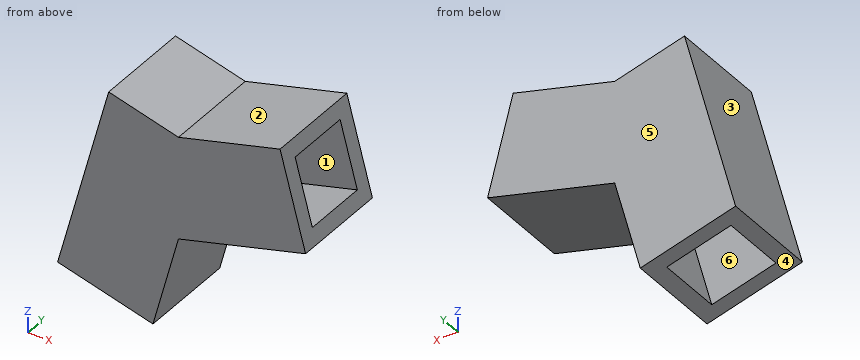
from build123d import *

# Parameters (mm, degrees)
BOSS_EXTRUDE1_DEPTH = 15
SKETCH2_W           = 10.1
SKETCH2_H           = 10.1
CUT_EXTRUDE1_DEPTH  = 18
SKETCH3_W           = 10.1
SKETCH3_H           = 10.1
CUT_EXTRUDE2_DEPTH  = 17
CUT_EXTRUDE3_REACH  = 41.336
SKETCH4_W           = 8
SKETCH4_H           = 8
CUT_EXTRUDE4_REACH  = 34.317
SKETCH5_W           = 8
SKETCH5_H           = 8
FILLET1_R           = 6
FILLET2_R           = 3


with BuildPart() as part:
    # Sketch1 → Boss-Extrude1 (new body)
    with BuildSketch(Plane(origin=(0, 0, 0), x_dir=(1, 0, 0), z_dir=(0, 1, 0))):
        Polygon((0, 0), (15.436230849, -4.13612559), (19.318516526, 10.352761804), (0, 15.529142706), (-3.882285677, 30.0180301), (-18.371173071, 26.135744424), (-10.606601718, -2.842030365), align=None)
    extrude(amount=BOSS_EXTRUDE1_DEPTH)

    # Sketch2 → Cut-Extrude1 (cut)
    with BuildSketch(Plane(origin=(15.436230849, 0, 4.13612559), x_dir=(0.2588190451025214, 0, -0.9659258262890681), z_dir=(0.9659258262890681, 0, 0.2588190451025214))):
        with Locations((7.5, 7.5)):
            Rectangle(SKETCH2_W, SKETCH2_H)
    extrude(amount=-CUT_EXTRUDE1_DEPTH, mode=Mode.SUBTRACT)

    # Sketch3 → Cut-Extrude2 (cut)
    with BuildSketch(Plane(origin=(-7.764571353, 0, -28.977774789), x_dir=(-0.9659258262890682, 0, 0.2588190451025212), z_dir=(-0.2588190451025212, 0, -0.9659258262890682))):
        with Locations((3.480762114, 7.5)):
            Rectangle(SKETCH3_W, SKETCH3_H)
    extrude(amount=-CUT_EXTRUDE2_DEPTH, mode=Mode.SUBTRACT)

    # Cut-Extrude3: up to this plane
    cut_extrude3_end = Plane(origin=(-11.60473103, 12.55, -10.349112038), z_dir=(-0.9659258262890682, 0, 0.2588190451025212))
    # Sketch4 → Cut-Extrude3 (cut, up to the surface)
    with BuildSketch(Plane(origin=(-1.950434024, 0, -0.522617222), x_dir=(0.25881904510252146, 0, -0.9659258262890681), z_dir=(0.9659258262890681, 0, 0.25881904510252146)), mode=Mode.PRIVATE) as cut_extrude3_sk1:
        with Locations((7.5, 7.5)):
            Rectangle(SKETCH4_W, SKETCH4_H)
    cut_extrude3_tool1 = split(extrude(cut_extrude3_sk1.sketch, amount=-CUT_EXTRUDE3_REACH, mode=Mode.PRIVATE), bisect_by=cut_extrude3_end, keep=Keep.BOTH, mode=Mode.PRIVATE)
    add(cut_extrude3_tool1.solids().sort_by_distance((-0.009291, 7.5, -7.767061))[0], mode=Mode.SUBTRACT)

    # Cut-Extrude4: up to this face of the body (flat: up to its plane)
    cut_extrude4_end = Plane(part.part.faces().sort_by_distance((-5.802700436, 7.5, -5.178295527))[0])
    # Sketch5 → Cut-Extrude4 (cut, up to the picked face)
    with BuildSketch(Plane(origin=(-3.364647586, 0, -12.557035742), x_dir=(-0.9659258262890682, 0, 0.25881904510252124), z_dir=(-0.25881904510252124, 0, -0.9659258262890682)), mode=Mode.PRIVATE) as cut_extrude4_sk1:
        with Locations((3.480762114, 7.5)):
            Rectangle(SKETCH5_W, SKETCH5_H)
    cut_extrude4_tool1 = split(extrude(cut_extrude4_sk1.sketch, amount=-CUT_EXTRUDE4_REACH, mode=Mode.PRIVATE), bisect_by=cut_extrude4_end, keep=Keep.BOTH, mode=Mode.PRIVATE)
    add(cut_extrude4_tool1.solids().sort_by(Axis((-6.726806, 7.5, -11.656148), (0.25881904510252124, 0, 0.9659258262890682)))[0], mode=Mode.SUBTRACT)

    # Fillet1
    fillet1_edges = [part.edges().sort_by_distance(p)[0] for p in [
        (-10.560833506, 7.5, -6.453233441),
    ]]
    fillet(fillet1_edges, radius=FILLET1_R)

    # Fillet2
    fillet2_edges = [part.edges().sort_by_distance(p)[0] for p in [
        (-11.531070004, 11.5, -10.074205347),
        (-0.915876519, 11.5, -12.151084448),
        (-0.915876519, 3.5, -12.151084448),
        (-11.531070004, 3.5, -10.074205347),
        (-4.129667829, 3.5, -4.730007791),
        (-9.904494707, 3.5, -7.109572239),
        (-4.129667829, 11.5, -4.730007791),
        (-9.904494707, 11.5, -7.109572239),
    ]]
    fillet(fillet2_edges, radius=FILLET2_R)


solid = part.part
Can you work these out from the model? Positions are in its coordinate system, mm. Face numbers are marked on the shaded views. A direction names the side the tool comes from. Coordinates: 2 decimals unless noted, no trailing zeros. Order: outer loops, then holes, each group sorted by start corner. A loop starts at its lowest first (then second) coordinate and runs counter-clockwise, first axis right, second up. Notation, with made-up numbers: (39, 37) -> (95, 37) arc R26 cw to (95, 64) -> close; hole circle Ø3 at (36.5, 54). An arc over 180 degrees is marked (long way). Use one line per item in the form item = value.
Q1. Imagine slicing it at C-C, the plane x = 4.5. List the corners of the cut face in (y, z) for me, then the cut area to 3 significant figures.
From the geometry:
outline = (0, -14.32) -> (15, -14.32) -> (15, 1.21) -> (0, 1.21) -> close; hole (2.45, -11.79) -> (12.55, -11.79) -> (12.55, -1.33) -> (2.45, -1.33) -> close
area = 127 mm²
Q2. Which directions (+Z, -Z, +X, -X, +Y, -Y) give clear straight access to the entire face, cutting with the end or side of a thin tool? Please do the marked faces 1, 2 and 3.
From the geometry:
face_1 = none
face_2 = +Z, +Y, -Y
face_3 = +Z, -X, +Y, -Y
Q3. Imagine slicing it at B-B, the plane y = 13.5. List the corners of the cut face in (x, z) for me, then the cut area to 3 significant figures.
From the geometry:
outline = (-18.37, -26.14) -> (-3.88, -30.02) -> (0, -15.53) -> (19.32, -10.35) -> (15.44, 4.14) -> (0, 0) -> (-10.61, 2.84) -> close
area = 690 mm²
Q4. Will these pins go through, and if not, where does the flat tip stop? P1, Ø15.5, axis at x = -6, z = -18.5, coming from the -Y side; P2, Ø3, axis at y = 3, z = -22.5, coming from the -X side; P3, Ø8, axis at y = 9, z = -11.5, coming from the -X side; P4, Ø4, axis at x = 5, y = 7, coming from the -Z side.
From the geometry:
P1 = 0
P2 = -17.8
P3 = -15.52
P4 = -14.73
Q5. Imagine slicing it at D-D, the plane z = -20.5. List the corners of the cut face in (x, y) for me.
From the geometry:
outline = (-16.86, 0) -> (-1.33, 0) -> (-1.33, 15) -> (-16.86, 15) -> close; hole (-14.32, 2.45) -> (-3.87, 2.45) -> (-3.87, 12.55) -> (-14.32, 12.55) -> close
Q6. I need wall thicknesses on L1, parallel to Y at x = 10, z = -5.5; L2, parallel to X at y = 5, z = -20; L3, parallel to Z at x = 6.5, y = 4. Which ranges of each line are inside material? Lowest first, please.
From the geometry:
L1 = 0 to 2.45, 12.55 to 15
L2 = -16.73 to -14.19, -3.73 to -1.2
L3 = -13.79 to -11.25, -0.79 to 1.74
Q7. We'd pull the mould along Y, two halves only. Please class the marked faces 4, 5 and 6: released by +Y, released by -Y, zero draft, split by the parting line, or undercut.
From the geometry:
face_4 = zero draft
face_5 = released by +Y
face_6 = undercut
